Part print with two shaded views. Sizes in mm from the minimum x, y, z corner. A direction names the side the tool comes from. Give positions to 0.01 mm unless a question says otherwise; leave off trailing zeros. Write each loop counter-clockwise with the first axis right and the second up, starting at its lowest first coordinate (ties: lowest second). Pieces come first, ordered by that corner, then holes. Notation, with made-up numbers: (49.25, 23) - (108.25, 23) arc R17 cw to (108.25, 51) - close; hole circle Ø4 at (59, 78). An arc over 180 degrees is marked (long way). Answer as a JSON object with one key per item and string values. Group by question number.
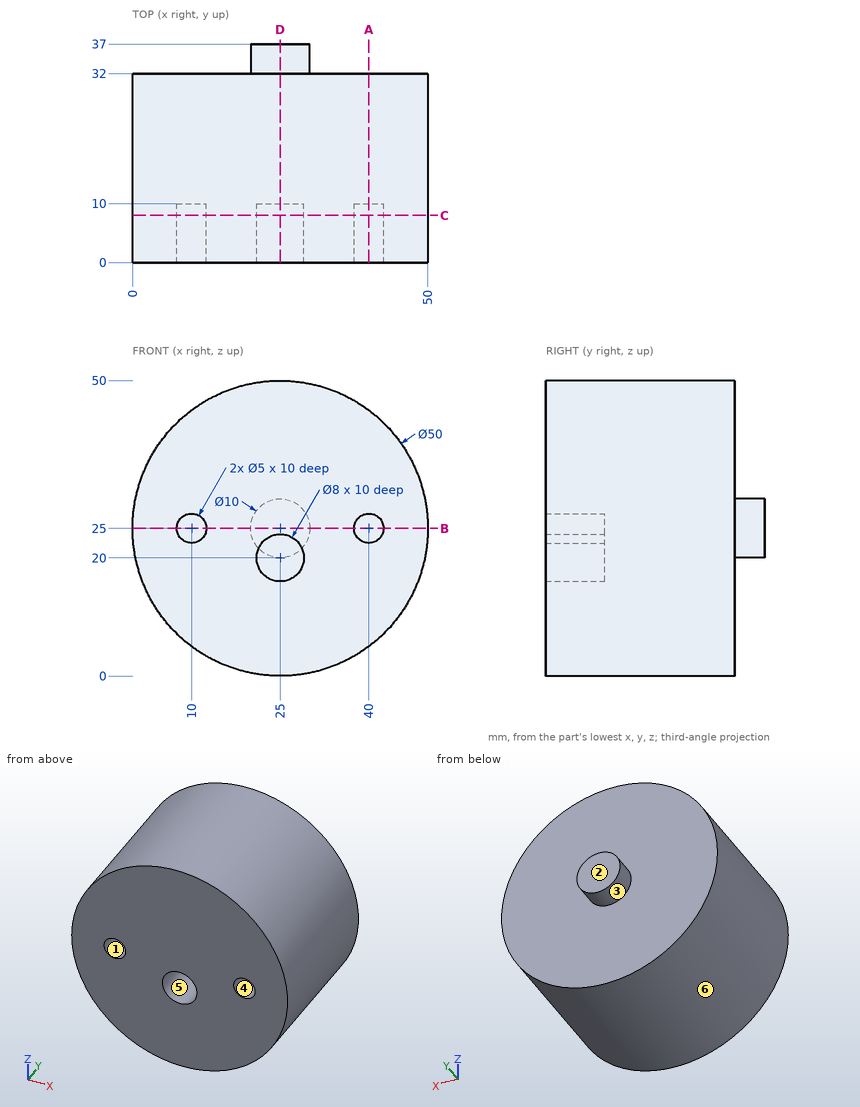
1) Drop flat-ended pins along their axis: P1, Ø1, axis at y = 27, z = 32, coming from the +X side; P2, Ø1, axis at y = 15.5, z = 22, coming from the +X side; P3, Ø2, axis at y = 15, z = 11.5, coming from the +X side. Give the stop position or say it passes through.
2) Saw through at A-A (x = 40). List the corners of the cut face in (y, z).
3) Two-plate mould, pull along Z, no slides. Class the marked faces 1, 2, 3 and 4: +Z half, -Z half, draft (parallel to the pull), parting line (faces both ways), or undercut.
4) Which spindle directions (+Z, -Z, +X, -X, +Y, -Y) get a long thin tool onto all of the face, cutting with end or side? Do the marked faces 5 and 6. Say none if no direction does.
5) Saw through at D-D (x = 25). List the corners of the cut face in (y, z).
6) Drill centre lines: line 1 along X through (y, z) = (6, 20); line 2 along Y through (x, z) = (40.5, 41); line 3 along Z through (x, y) = (40, 6.25). Where is each one in solid material? Low to high. Write a range as from..to.
7) Saw through at C-C (y = 8). List the corners of the cut face in (x, z), and give its area (3 significant figures).
8) Saw through at B-B (z = 25). List the corners of the cut face in (x, y).
Checks:
{
 "1": {"P1": "x = 49.14", "P2": "x = 49.87", "P3": "x = 46.65"},
 "2": {"outline": "(0, 5) - (32, 5) - (32, 45) - (0, 45) - (0, 27.5) - (10, 27.5) - (10, 22.5) - (0, 22.5) - close"},
 "3": {"face 1": "undercut", "face 2": "draft", "face 3": "parting line", "face 4": "undercut"},
 "4": {"face 5": "-Y", "face 6": "+Y, -Y"},
 "5": {"outline": "(0, 0) - (32, 0) - (32, 20) - (37, 20) - (37, 30) - (32, 30) - (32, 50) - (0, 50) - (0, 24) - (10, 24) - (10, 16) - (0, 16) - close"},
 "6": {"line 1": "0.51..21, 29..49.49", "line 2": "0..32", "line 3": "5..22.5, 27.5..45"},
 "7": {"outline": "circle Ø50 at (25, 25); hole circle Ø5 at (10, 25); hole circle Ø8 at (25, 20); hole circle Ø5 at (40, 25)", "area": "1,870 mm2"},
 "8": {"outline": "(0, 0) - (7.5, 0) - (7.5, 10) - (12.5, 10) - (12.5, 0) - (37.5, 0) - (37.5, 10) - (42.5, 10) - (42.5, 0) - (50, 0) - (50, 32) - (30, 32) - (30, 37) - (20, 37) - (20, 32) - (0, 32) - close"}
}
